from build123d import *

# Parameters (mm, degrees)
F0_W     = 25.4
F0_H     = 25.4
F1_DEPTH = 25.4
F2_T     = -2.54


with BuildPart() as f1:
    # F0 (on Front) → F1 (new body)
    with BuildSketch(Plane.XZ):
        Rectangle(F0_W, F0_H)
    extrude(amount=F1_DEPTH)

    # F2
    f2_openings = [f1.faces().sort_by_distance(p)[0] for p in [
        (0, -12.7, 12.7),
    ]]
    offset(amount=F2_T, openings=f2_openings)


with BuildPart() as f3_1:
    # F3: copy of F1
    add(f1.part)


solid = f1.part
Can you work these out from the model? Positions are in its coordinate system, mm. A direction names the side the tool comes from. Coordinates: 2 decimals unless noted, no trailing zeros. Order: outer loops, then holes, each group sorted by start corner. A loop starts at its lowest first (then second) coordinate and runs counter-clockwise, first axis right, second up. Notation, with made-up numbers: (86, 8) - (131, 8) arc R30 ccw to (131, 33) - close; hole circle Ø3 at (-22, 89.25). An arc over 180 degrees is marked (long way). Answer as a JSON object with one key per item and string values. Group by question number.
Q1. We'd pull the mould along Y, two halves only. Please class faces 1 (the face through (0, -13, -10.16)), 2 (the face through (0, 0, 0)), 3 (the face through (0, -25.4, 0)): +Y half, -Y half, draft (parallel to the pull), parting line (faces both ways), or undercut.
Q2. I need wall thicknesses on line 1 (Y direction, x = 1.75, z = -1.5); line 2 (X direction, y = -15.5, z = -3.5); line 3 (Z direction, x = 3.5, y = -2.75). Which ranges of each line are inside material? Lowest first, please. Write a range as from..to.
Q3. Will these pins go through, and if not, where does the flat tip stop? P1, Ø3, axis at x = -2, y = -22, coming from the +Z side; P2, Ø6, axis at x = -3, y = -17.5, coming from the +Z side.
Q4. Imagine slicing it at B-B (x = 1). Please give me the cut outline in (y, z), and give its area (3 significant figures).
Q5. Imagine slicing it at C-C (y = -9.25). Please give me the cut outline in (x, z), and give its area (3 significant figures).
Q6. On a 3-axis mill with a long thin cutter (end or side, diameter ignored), from which of +Z, -Z, +X, -X, +Y, -Y can I reach the whole of each face in a straight line? I mean faces 4 (the face through (0, -22.86, 1)), 5 (the face through (0, -13, -12.7)). Say none if no direction works.
Q7. Imagine slicing it at A-A (z = 10). Please give me the cut outline in (x, y), and give its area (3 significant figures).
Determined:
{
 "1": {"face 1": "undercut", "face 2": "+Y half", "face 3": "-Y half"},
 "2": {"line 1": "y = -25.4..-22.86, -2.54..0", "line 2": "x = -12.7..-10.16, 10.16..12.7", "line 3": "z = -12.7..-10.16"},
 "3": {"P1": "stops at z = 12.7", "P2": "stops at z = -10.16"},
 "4": {"outline": "(-25.4, -12.7) - (0, -12.7) - (0, 12.7) - (-2.54, 12.7) - (-2.54, -10.16) - (-22.86, -10.16) - (-22.86, 12.7) - (-25.4, 12.7) - close", "area": "181 mm2"},
 "5": {"outline": "(-12.7, -12.7) - (12.7, -12.7) - (12.7, 12.7) - (10.16, 12.7) - (10.16, -10.16) - (-10.16, -10.16) - (-10.16, 12.7) - (-12.7, 12.7) - close", "area": "181 mm2"},
 "6": {"face 4": "+Z", "face 5": "-Z, +X, -X, +Y, -Y"},
 "7": {"outline": "(-12.7, -25.4) - (12.7, -25.4) - (12.7, 0) - (-12.7, 0) - close; hole (-10.16, -22.86) - (10.16, -22.86) - (10.16, -2.54) - (-10.16, -2.54) - close", "area": "232 mm2"}
}
